Here's the drawing with two shaded views (mm, measured from the low corner). I have some questions. Coordinates: 2 decimals unless noted, no trailing zeros. Order: outer loops, then holes, each group sorted by start corner. A loop starts at its lowest first (then second) coordinate and runs counter-clockwise, first axis right, second up. Notation, with made-up numbers: (71.25, 44.25) -> (85.25, 44.25) arc R14 ccw to (85.25, 48.25) -> close; hole circle Ø7 at (1, -32.75). An arc over 180 degrees is marked (long way). Answer as a JSON object with one key per item and string values. Group by question number.
(1) I want a section at B-B, the plane x = 44. List the corners of the cut face in (y, z) for me (1 decimal).
(2) I want a section at A-A, the plane z = 29.5. List the corners of the cut face in (x, y) for me (1 decimal).
(3) For pin 1 (5 mm diameter, centred on x = 4, y = 20.5, fed in from +Z); pin 2 (7.5 mm diameter, centred on x = 478.5, y = 24.5, fed in from -Z); pin 3 (2 mm diameter, centred on y = 168.5, z = 62, fed in from -X); pin 4 (5 mm diameter, centred on x = 96.5, z = 35, fed in from -Y) (1 decimal), each with a flat end and sliding along its axis, tell me the tip position at first contact or that it passes through.
(4) If we mould it in two halves opening along X, with no side actions, what happens to the marked faces 1, 2 and 3? For each: pulls with the +X half, pulls with the -X half, needs draft (parallel to the pull), parting line crosses it, or undercut.
(5) I need wall thicknesses on line 1 (Y direction, x = 134, z = 81.5) (1 decimal). Which ranges of the line are inside material? Lowest first, please.
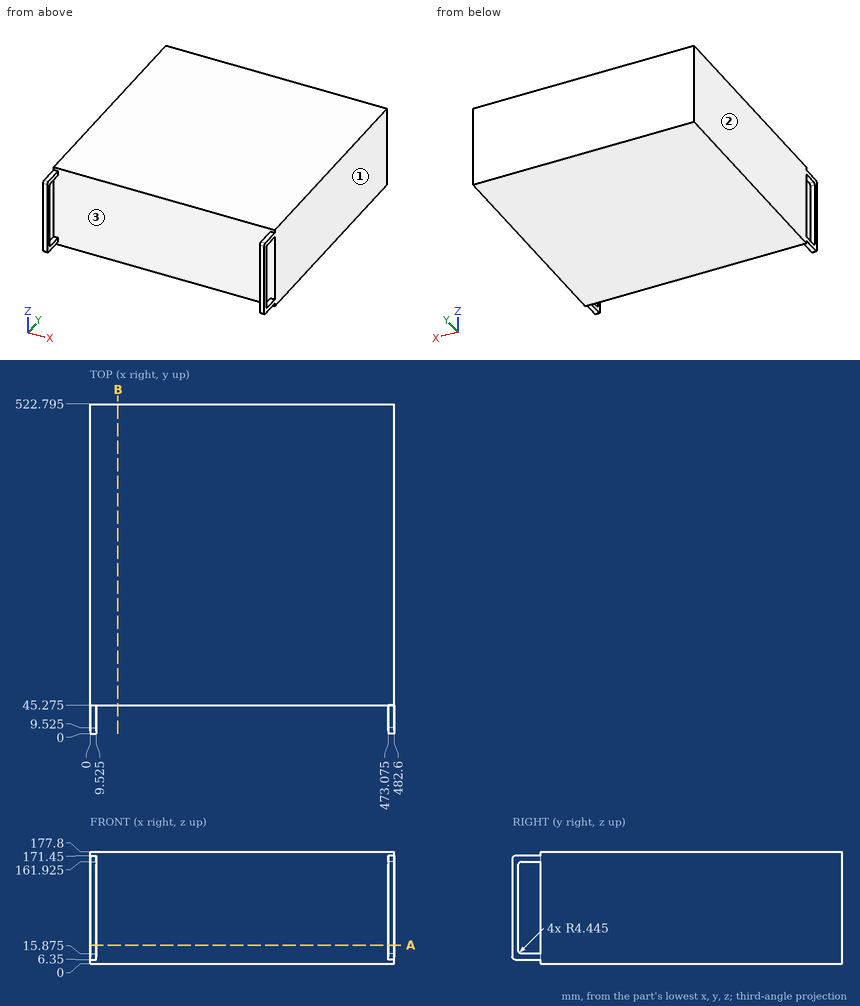
Computed values:
{
 "1": {"outline": "(45.3, 0) -> (522.8, 0) -> (522.8, 177.8) -> (45.3, 177.8) -> close"},
 "2": {"outline": "(0, 0) -> (9.5, 0) -> (9.5, 9.5) -> (0, 9.5) -> close; (0, 45.3) -> (482.6, 45.3) -> (482.6, 522.8) -> (0, 522.8) -> close; (473.1, 0) -> (482.6, 0) -> (482.6, 9.5) -> (473.1, 9.5) -> close"},
 "3": {"pin 1": "stops at z = 171.45", "pin 2": "stops at z = 6.35", "pin 3": "stops at x = 0", "pin 4": "stops at y = 45.3"},
 "4": {"face 1": "pulls with the +X half", "face 2": "pulls with the -X half", "face 3": "undercut"},
 "5": {"line 1": "y = 45.3 to 522.8"}
}
